```python
from build123d import *

# Parameters (mm, degrees)
F1_DEPTH = 3
F3_DEPTH = 3
F4_DEPTH = 3


with BuildPart() as f1:
    # F0 (on Front) → F1 (new body)
    with BuildSketch(Plane.XZ):
        with BuildLine():
            ThreePointArc((10.610182, -21.472413), (9.43467, -23.817103), (8.162286, -26.110668))
            ThreePointArc((8.162286, -26.110668), (4.736187, -40.380972), (8.162286, -54.651275))
            ThreePointArc((8.162286, -54.651275), (16.377217, -63.246062), (24.791062, -71.646221))
            ThreePointArc((24.791062, -71.646221), (26.102479, -75.930715), (26.647892, -80.3781))
            ThreePointArc((26.647892, -80.3781), (31.515082, -83.360934), (37.148613, -84.282979))
            ThreePointArc((37.148613, -84.282979), (42.081838, -83.311469), (46.856795, -81.736565))
            ThreePointArc((46.856795, -81.736565), (47.86306, -76.886336), (48.831385, -72.028391))
            ThreePointArc((48.831385, -72.028391), (55.688335, -64.651002), (63.137703, -57.872318))
            ThreePointArc((63.137703, -57.872318), (69.428725, -39.743128), (63.137703, -21.613939))
            ThreePointArc((63.137703, -21.613939), (62.345878, -7.148671), (48.831385, -12.366854))
            ThreePointArc((48.831385, -12.366854), (36.569551, -10.876763), (24.25742, -11.868899))
            ThreePointArc((24.25742, -11.868899), (11.154848, -7.747843), (10.610182, -21.472413))
        make_face()
    extrude(amount=F1_DEPTH)

    # F2 (on face) → F3 (join)
    with BuildSketch(Plane.XZ.offset(3)):
        with BuildLine():
            ThreePointArc((22.065133, -61.21042), (26.430602, -68.396115), (28.142098, -76.627903))
            ThreePointArc((28.142098, -76.627903), (37.20821, -76.271267), (46.260461, -76.886336))
            ThreePointArc((46.260461, -76.886336), (47.153606, -68.266964), (52.337427, -61.322954))
            ThreePointArc((52.337427, -61.322954), (50.114304, -61.50095), (47.903072, -61.21042))
            ThreePointArc((47.903072, -61.21042), (46.555062, -64.457231), (43.912064, -66.775307))
            ThreePointArc((43.912064, -66.775307), (44.722613, -62.717523), (44.03321, -58.637409))
            ThreePointArc((44.03321, -58.637409), (40.671762, -57.546974), (37.148613, -57.271644))
            ThreePointArc((37.148613, -57.271644), (33.581827, -57.670054), (30.184889, -58.828287))
            ThreePointArc((30.184889, -58.828287), (29.6759, -62.863739), (30.266298, -66.888086))
            ThreePointArc((30.266298, -66.888086), (27.649068, -64.531266), (26.475836, -61.21042))
            ThreePointArc((26.475836, -61.21042), (24.270484, -61.623817), (22.065133, -61.21042))
        make_face()
        with BuildLine():
            Line((32.305945, -74.377179), (30.617898, -69.65065))
            ThreePointArc((30.617898, -69.65065), (33.670475, -72.046287), (37.148613, -70.325866))
            ThreePointArc((37.148613, -70.325866), (41.008138, -71.808616), (44.129851, -69.097642))
            Line((44.129851, -69.097642), (42.557646, -73.926551))
            Line((42.557646, -73.926551), (32.305945, -74.377179))
        make_face(mode=Mode.SUBTRACT)
        with BuildLine():
            ThreePointArc((30.184889, -58.828287), (28.250667, -59.895266), (26.475836, -61.21042))
            ThreePointArc((26.475836, -61.21042), (27.649068, -64.531266), (30.266298, -66.888086))
            ThreePointArc((30.266298, -66.888086), (29.6759, -62.863739), (30.184889, -58.828287))
        make_face()
        with BuildLine():
            ThreePointArc((43.912064, -66.775307), (46.555062, -64.457231), (47.903072, -61.21042))
            ThreePointArc((47.903072, -61.21042), (46.068198, -59.773426), (44.03321, -58.637409))
            ThreePointArc((44.03321, -58.637409), (44.722613, -62.717523), (43.912064, -66.775307))
        make_face()
    extrude(amount=F3_DEPTH)

    # F2 (on face) → F4 (join)
    with BuildSketch(Plane.XZ.offset(3)):
        with BuildLine():
            ThreePointArc((22.065133, -61.21042), (26.430602, -68.396115), (28.142098, -76.627903))
            ThreePointArc((28.142098, -76.627903), (37.20821, -76.271267), (46.260461, -76.886336))
            ThreePointArc((46.260461, -76.886336), (47.153606, -68.266964), (52.337427, -61.322954))
            ThreePointArc((52.337427, -61.322954), (50.114304, -61.50095), (47.903072, -61.21042))
            ThreePointArc((47.903072, -61.21042), (46.555062, -64.457231), (43.912064, -66.775307))
            ThreePointArc((43.912064, -66.775307), (44.722613, -62.717523), (44.03321, -58.637409))
            ThreePointArc((44.03321, -58.637409), (40.671762, -57.546974), (37.148613, -57.271644))
            ThreePointArc((37.148613, -57.271644), (33.581827, -57.670054), (30.184889, -58.828287))
            ThreePointArc((30.184889, -58.828287), (29.6759, -62.863739), (30.266298, -66.888086))
            ThreePointArc((30.266298, -66.888086), (27.649068, -64.531266), (26.475836, -61.21042))
            ThreePointArc((26.475836, -61.21042), (24.270484, -61.623817), (22.065133, -61.21042))
        make_face()
        with BuildLine():
            Line((32.305945, -74.377179), (30.617898, -69.65065))
            ThreePointArc((30.617898, -69.65065), (33.670475, -72.046287), (37.148613, -70.325866))
            ThreePointArc((37.148613, -70.325866), (41.008138, -71.808616), (44.129851, -69.097642))
            Line((44.129851, -69.097642), (42.557646, -73.926551))
            Line((42.557646, -73.926551), (32.305945, -74.377179))
        make_face(mode=Mode.SUBTRACT)
        with BuildLine():
            ThreePointArc((30.184889, -58.828287), (28.250667, -59.895266), (26.475836, -61.21042))
            ThreePointArc((26.475836, -61.21042), (27.649068, -64.531266), (30.266298, -66.888086))
            ThreePointArc((30.266298, -66.888086), (29.6759, -62.863739), (30.184889, -58.828287))
        make_face()
        with BuildLine():
            ThreePointArc((43.912064, -66.775307), (46.555062, -64.457231), (47.903072, -61.21042))
            ThreePointArc((47.903072, -61.21042), (46.068198, -59.773426), (44.03321, -58.637409))
            ThreePointArc((44.03321, -58.637409), (44.722613, -62.717523), (43.912064, -66.775307))
        make_face()
    extrude(amount=F4_DEPTH)


solid = f1.part
```
Check sheet for the modelled part. Datum: model origin and axes. Units: mm. A direction names the side the tool comes from. Round coordinates to 2 decimals unless told otherwise and drop trailing zeros. Loops run counter-clockwise (first coordinate to the right, second up) from the corner with the lowest first, then second, coordinate; pieces in that order, holes last. Notation, with made-up numbers: (-38.75, -23.75) - (14.25, -23.75) arc R29 cw to (14.25, 12.25) - close; hole circle Ø8 at (13.5, 74). An arc over 180 degrees is marked (long way). Answer as a JSON object with one key per item and string values. Group by question number.
Q1. Sectioned sample at B-B, the plane y = -4.3. Enter the section's corners in (x, z), plus the area to 3 significant figures.
Q2. Sectioned sample at C-C, the plane z = -73. Enter the section's corners in (x, y) (3 decimals), plus the area to 3 significant figures.
Q3. Sectioned sample at A-A, the plane x = 64. Enter the section's corners in (y, z).
Q4. Scan lines: line 1 along Y through (x, z) = (48, -56); line 2 along Z through (x, y) = (40, -3.5); line 3 along X through (y, z) = (-2.15, -60). Record each from-to range of solid material in increasing order. Write a range as [from, to].
Q5. Sectioned sample at D-D, the plane x = 34. Enter the section's corners in (y, z).
Q6. Mould release check, pull along Z, two halves, no side actions. Record for faces 1 (the face through (33.61, -4.48, -72.04)), 2 (the face through (37, 0, -44)), 3 (the face through (16.261, -1.479, -63.127)): released by +Z, released by -Z, zero draft, split by the parting line, or undercut.
Q7. Set-up check for faces 4 (the face through (9.452, -1.479, -23.785)), 5 (the face through (37.5, -4.48, -74.15)), 6 (the face through (47.11, -4.48, -68.38)): record each of +Z, -Z, +X, -X, +Y, -Y from which the full face is reachable in a straight line by a thin tool's end or side.
Q8. Gauge pin test, flat ends, axial feed: P1, Ø3, axis at y = -2, z = -73.5, coming from the -X side; P2, Ø2, axis at y = -1, z = -19.5, coming from the -X side; P3, Ø1.5, axis at x = 35.5, y = -1, coming from the +Z side. Record the tip position at first contact, or that the pin passes through.
Solution:
{
 "1": {"outline": "(22.07, -61.21) arc R24.78 cw to (28.14, -76.63) arc R84.71 cw to (46.26, -76.89) arc R16.3 cw to (52.34, -61.32) arc R10.61 cw to (47.9, -61.21) arc R15.03 ccw to (44.03, -58.64) arc R15.03 ccw to (37.15, -57.27) arc R16.54 ccw to (30.18, -58.83) arc R16.54 ccw to (26.48, -61.21) arc R6.09 cw to start; hole (30.62, -69.65) - (32.31, -74.38) - (42.56, -73.93) - (44.13, -69.1) arc R4.01 cw to (37.15, -70.33) arc R3.64 cw to start", "area": "355 mm²"},
 "2": {"outline": "(25.295, -3) - (27.748, -3) - (27.748, -6) - (31.814, -6) - (31.814, -3) - (42.859, -3) - (42.859, -6) - (46.081, -6) - (46.081, -3) - (48.641, -3) - (48.641, 0) - (25.295, 0) - close", "area": "91.9 mm²"},
 "3": {"outline": "(-3, -56.72) - (0, -56.72) - (0, -22.76) - (-3, -22.76) - close; (-3, -20.81) - (0, -20.81) - (0, -8.53) - (-3, -8.53) - close"},
 "4": {"line 1": "y = [-3, 0]", "line 2": "z = [-76.36, -74.04], [-71.86, -57.43]", "line 3": "x = [13.23, 60.66]"},
 "5": {"outline": "(-6, -76.29) - (-3, -76.29) - (-3, -84.05) - (0, -84.05) - (0, -10.88) - (-3, -10.88) - (-3, -57.58) - (-6, -57.58) - (-6, -72.07) - (-3, -72.07) - (-3, -74.3) - (-6, -74.3) - close"},
 "6": {"face 1": "undercut", "face 2": "zero draft", "face 3": "released by -Z"},
 "7": {"face 4": "-X, +Y, -Y", "face 5": "-Y", "face 6": "+X, -Y"},
 "8": {"P1": "stops at x = 24.93", "P2": "stops at x = 8.31", "P3": "stops at z = -10.86"}
}
